```python
from build123d import *

# Parameters (mm, degrees)
MODEL_R           = 1.4
MODEL_R_2         = 1
BRIDA_BASE1_DEPTH = 1


# Sheet-metal steps are written as plain solids
with BuildPart() as part:
    # Model → Brida base1 (new body)
    with BuildSketch(Plane.XY):
        with BuildLine():
            Line((40.2059904, -5.7615616), (42.197855138, 22.819737764))
            ThreePointArc((42.197855138, 22.819737764), (44.604363348, 38.449201588), (47.010871557, 22.819737764))
            Line((47.010871557, 22.819737764), (50.2059904, -5.7615616))
            Line((50.2059904, -5.7615616), (50.2059904, -15.7615616))
            ThreePointArc((50.2059904, -15.7615616), (45.2059904, -20.7615616), (40.2059904, -15.7615616))
            Line((40.2059904, -15.7615616), (40.2059904, -5.7615616))
        make_face()
        with Locations((45.2059904, -15.7615616)):
            Circle(MODEL_R, mode=Mode.SUBTRACT)
        with Locations((45.2059904, -3.2615616)):
            Circle(MODEL_R_2, mode=Mode.SUBTRACT)
    extrude(amount=-BRIDA_BASE1_DEPTH)


solid = part.part
```
Source: CAD feature listing. Evaluate the final solid. Frame: model axes, mm. A direction names the side the tool comes from. Give positions to 0.01 mm unless a question says otherwise; leave off trailing zeros. Write each loop counter-clockwise with the first axis right and the second up, starting at its lowest first coordinate (ties: lowest second). Pieces come first, ordered by that corner, then holes.
1. Section query A-A (x = 49). Return the cut outline in (y, z), then the cut area to 3 significant figures.
2. Section query C-C (z = -0.15). Return the cut outline in (x, y).
3. Access query for faces 5 (the face through (45.32, -20.76, -0.49)), 6 (the face through (44.207, -3.218, -0.493)), 7 (the face through (50.206, -10.7, -0.5)), 8 (the face through (41.19, 8.33, -0.49)), 9 (the face through (40.206, -10.8, -0.5)). Directions: +Z, -Z, +X, -X, +Y, -Y. A direction counts if a zero-diameter tool reaches every point of the face in a straight line with its end or side. Return the directions, or none.
4. First-contact query: pin 1 (0.5 mm diameter, centred on y = -10.5, z = -0.5, fed in from +X); pin 2 (2 mm diameter, centred on x = 38.5, y = 10, fed in from -Z). Flat tips, straight axial feed; report the tip coordinate or a pass-through.
5. Section query D-D (y = -11). Return the cut outline in (x, z), then the cut area to 3 significant figures.
6. Section query B-B (x = 45). Return the cut outline in (y, z), then the cut area to 3 significant figures.
7. Pull-direction query (X, two-part tool) for faces 1 (the face through (44.09, -16.61, -0.49)), 2 (the face through (44.287, 38.443, -0.493)), 3 (the face through (48.586, 8.729, -0.493)), 4 (the face through (45, 9, -1)); classes: +X half, -X half, draft (parallel to the pull), parting line (faces both ways), or undercut.
8. Material intervals for line 1 along Y through (x, z) = (44.75, -0.85); line 2 along X through (y, z) = (-10.5, -0.8); line 3 along X through (y, z) = (19, -0.85), sorted ascending.
Output values:
1. outline: (-19.02, -1) - (5.03, -1) - (5.03, 0) - (-19.02, 0) - close; (23.77, -1) - (37.13, -1) - (37.13, 0) - (23.77, 0) - close
1. area: 37.4 mm2
2. outline: (40.21, -15.76) arc R5 ccw to (50.21, -15.76) - (50.21, -5.76) - (47.01, 22.82) arc R8 ccw (long way) to (42.2, 22.82) - (40.21, -5.76) - close; hole circle Ø2.8 at (45.21, -15.76); hole circle Ø2 at (45.21, -3.26)
3. face 5: +Z, -Z, -Y
3. face 6: +Z, -Z
3. face 7: +Z, -Z, +X, -Y
3. face 8: +Z, -Z, -X
3. face 9: +Z, -Z, -X, -Y
4. pin 1: stops at x = 50.21
4. pin 2: passes through
5. outline: (40.21, -1) - (50.21, -1) - (50.21, 0) - (40.21, 0) - close
5. area: 10.0 mm2
6. outline: (-20.76, -1) - (-17.15, -1) - (-17.15, 0) - (-20.76, 0) - close; (-14.38, -1) - (-4.24, -1) - (-4.24, 0) - (-14.38, 0) - close; (-2.28, -1) - (38.44, -1) - (38.44, 0) - (-2.28, 0) - close
6. area: 54.5 mm2
7. face 1: undercut
7. face 2: parting line
7. face 3: +X half
7. face 4: draft
8. line 1: y = -20.74 to -17.09, -14.44 to -4.15, -2.37 to 38.45
8. line 2: x = 40.21 to 50.21
8. line 3: x = 41.93 to 47.44
